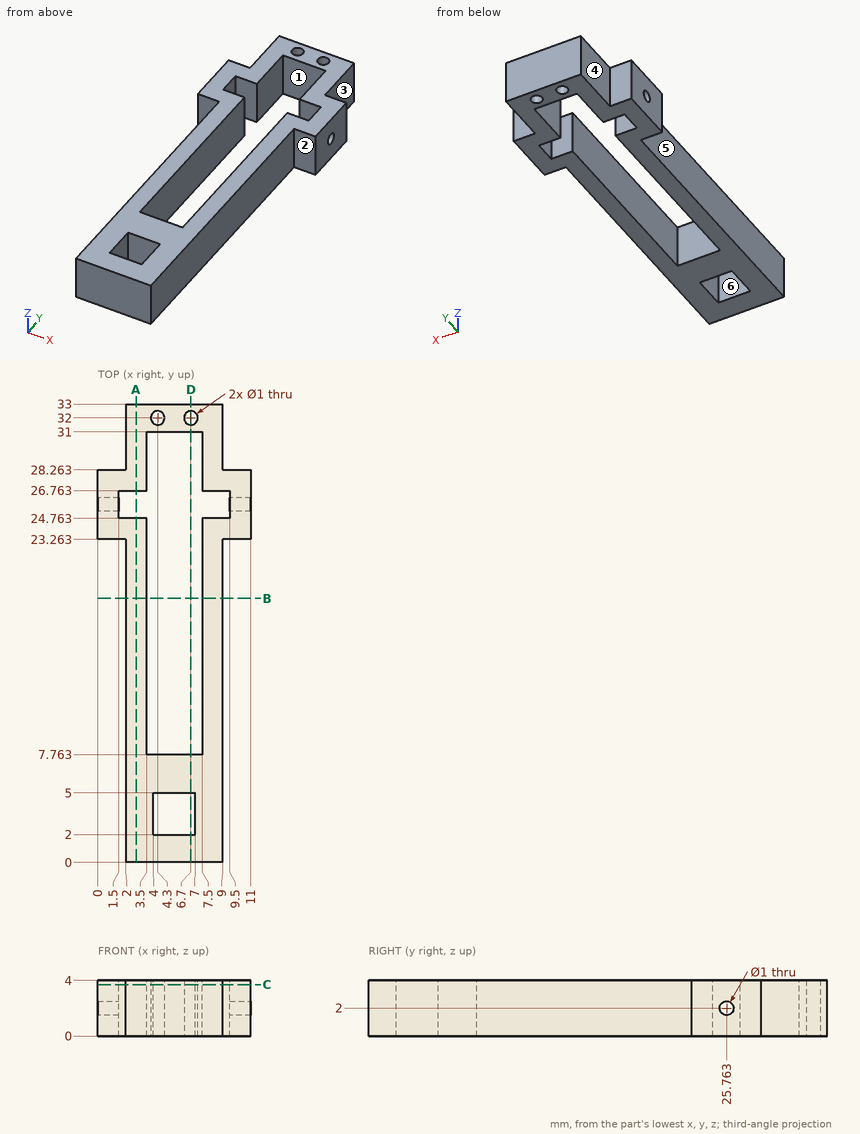
The drawing under review shows one solid part. Ordinate dimensions are in mm from its lowest x, y, z. A direction names the side the tool comes from. Round coordinates to 2 decimals unless told otherwise and drop trailing zeros. Loops run counter-clockwise (first coordinate to the right, second up) from the corner with the lowest first, then second, coordinate; pieces in that order, holes last. Notation, with made-up numbers: (18, -16.75) - (25, -16.75) arc R27 cw to (25, 19.25) - close; hole circle Ø4 at (70, 61.25). An arc over 180 degrees is marked (long way). Use a Markdown table: item, result. Add a question column.
Q1. For probe 1 along Y at (x, z) = (4.3, 1.4); probe 2 along X at (y, z) = (32, 2.05); probe 3 along Y at (x, z) = (10.5, 2), list the stretches that pass through material, from the lowest coordinate up.
Q2. Add section C-C (z = 3.7). State how many separate pieces and enclosed holes the cut face has.
Q3. Insertion check: pin 1 Ø2 at (y, z) = (17, 1) entering from -X; pin 2 Ø1.6 at (x, z) = (10, 2.5) entering from +Y; pin 3 Ø1.5 at (y, z) = (3, 1.5) entering from +X. Each pin has a flat end and moves straight along its axis. Give the tip position at first contact, or say it passes through.
Q4. Add section A-A (x = 2.75). State the section outline as (y, z) points.
Q5. Machinability: for the marked faces 4, 5 and 6, which of the approach directions +Z, -Z, +X, -X, +Y, -Y give a long, thin tool a straight path to every point of the face, cutting with its end or side? Answer none if there is none.
Q6. Add section D-D (x = 6.7). State the section outline as (y, z) points.
Q7. The part is to be moulded in two halves that separate along Y. For the marked faces 1, 2 and 3, say which applies: pulls with the +Y half, pulls with the -Y half, needs draft (parallel to the pull), parting line crosses it, or undercut.
Q8. Add section B-B (y = 19). State the section outline as (x, z) points, plus the area to 3 significant figures.
Worked answers:
| question | item | result |
|---|---|---|
| 1 | probe 1 | 0 to 2, 5 to 7.76, 31 to 31.5, 32.5 to 33 |
| 1 | probe 2 | 2 to 3.8, 4.8 to 6.2, 7.2 to 9 |
| 1 | probe 3 | 23.26 to 25.26, 26.26 to 28.26 |
| 2 | separate pieces | 1 |
| 2 | enclosed holes | 4 |
| 3 | pin 1 | x = 2 |
| 3 | pin 2 | y = 28.26 |
| 3 | pin 3 | x = 9 |
| 4 | outline | (0, 0) - (24.76, 0) - (24.76, 4) - (0, 4) - close; (26.76, 0) - (33, 0) - (33, 4) - (26.76, 4) - close |
| 5 | face 4 | +Z, -Z, -X, +Y |
| 5 | face 5 | +Z, -Z, -X, -Y |
| 5 | face 6 | +Z, -Z |
| 6 | outline | (0, 0) - (2, 0) - (2, 4) - (0, 4) - close; (5, 0) - (7.76, 0) - (7.76, 4) - (5, 4) - close; (31, 0) - (31.5, 0) - (31.5, 4) - (31, 4) - close; (32.5, 0) - (33, 0) - (33, 4) - (32.5, 4) - close |
| 7 | face 1 | undercut |
| 7 | face 2 | pulls with the -Y half |
| 7 | face 3 | needs draft |
| 8 | outline | (2, 0) - (3.5, 0) - (3.5, 4) - (2, 4) - close; (7.5, 0) - (9, 0) - (9, 4) - (7.5, 4) - close |
| 8 | area | 12.0 mm² |
